Geometry check sheet. Reference: the model listing, model coordinates, mm. A direction names the side the tool comes from. Give positions to 0.01 mm unless a question says otherwise; leave off trailing zeros. Write each loop counter-clockwise with the first axis right and the second up, starting at its lowest first coordinate (ties: lowest second). Pieces come first, ordered by that corner, then holes. Notation, with made-up numbers: (48.25, 43.25) - (81.25, 43.25) arc R18 ccw to (81.25, 69.25) - close; hole circle Ø8 at (27.25, 29). An arc over 180 degrees is marked (long way). Write item = value, one per line. Start each with the question number.
(1) Section check C-C, the plane x = -46. Enter the section's corners in (y, z).
(2) Section check A-A, the plane y = 31.5. Enter the section's corners in (x, z).
(3) Section check D-D, the plane y = 37.5. Enter the section's corners in (x, z), plus the area to 3 significant figures.
(4) Section check B-B, the plane z = 2.65. Enter the section's corners in (x, y), plus the area to 3 significant figures.
(5) Depth check by flat-ended pin: pin 1 Ø1 at (y, z) = (36.5, 1) entering from -X; pin 2 Ø3 at (x, y) = (-38.33, 34.29) entering from +Z; pin 3 Ø1 at (x, z) = (-39.5, 3.5) entering from +Y. Enter the tip coordinate at first touch or a pass-through.
(6) Thickness scan on L1, parallel to X at y = 32.75, z = 2.05; L2, parallel to X at y = 33.25, z = 2.8; L3, parallel to Z at x = -35.5, y = 36.25. Record the ranges inside material, lowest first.
(7) Access from +Z, -Z, +X, -X, +Y, -Y to the whole of each face (thin tool, end or side, straight path). Record for faces 1 (the flat face through (-43, 34, 0)), 2 (the flat face through (-38, 34, 1)).
(8) Draft check along X on faces 3 (the cylindrical face through (-49.21, 32.47, 2.97)), 4 (the flat face through (-46, 32, 5)). Enter one of: pulls with the +X half, pulls with the -X half, needs draft (parallel to the pull), parting line crosses it, or undercut.
```python
from build123d import *

# Parameters (mm, degrees)
F0_R     = 3
F0_R_2   = 2
F1_DEPTH = 5
F2_DEPTH = 1
F3_DEPTH = 0.5


# Not quite as in the source:
# - a feature names something its author has since deleted; it is built from what else it names


with BuildPart() as f1:
    # F0 (on Top) → F1 (new body)
    with BuildSketch(Plane.XY):
        with Locations((-46.8270219862, 34.2949032784)):
            Circle(F0_R)
        with Locations((-46.8270219862, 34.2949032784)):
            Circle(F0_R_2, mode=Mode.SUBTRACT)
    extrude(amount=F1_DEPTH)

    # F0 (on Top) → F2 (join)
    with BuildSketch(Plane.XY):
        with BuildLine():
            ThreePointArc((-42.8347911995, 34.0457179145), (-42.8289647614, 34.1702500531), (-42.8270219862, 34.2949032784))
            ThreePointArc((-42.8270219862, 34.2949032784), (-42.8289647614, 34.4195565036), (-42.8347911995, 34.5440886422))
            ThreePointArc((-42.8347911995, 34.5440886422), (-50.8270219862, 34.2949032784), (-42.8347911995, 34.0457179145))
        make_face()
        with Locations((-46.8270219862, 34.2949032784)):
            Circle(F0_R, mode=Mode.SUBTRACT)
        with Locations((-46.8270219862, 34.2949032784)):
            Circle(F0_R_2)
    extrude(amount=F2_DEPTH)



with BuildPart() as f1b:
    # F0 (on Top) → F1, piece 2 (new body)
    with BuildSketch(Plane.XY):
        with Locations((-38.3270219862, 34.2949032784)):
            Circle(F0_R)
        with Locations((-38.3270219862, 34.2949032784)):
            Circle(F0_R_2, mode=Mode.SUBTRACT)
    extrude(amount=F1_DEPTH)

    # F0 (on Top) → F2, piece 2 (join)
    with BuildSketch(Plane.XY):
        with BuildLine():
            ThreePointArc((-34.3270219862, 34.2949032784), (-38.202368761, 38.2929605032), (-42.319252773, 34.5440886422))
            ThreePointArc((-42.319252773, 34.5440886422), (-42.3270219862, 34.2949032784), (-42.319252773, 34.0457179145))
            ThreePointArc((-42.319252773, 34.0457179145), (-38.202368761, 30.2968460535), (-34.3270219862, 34.2949032784))
        make_face()
        with Locations((-38.3270219862, 34.2949032784)):
            Circle(F0_R, mode=Mode.SUBTRACT)
        with Locations((-38.3270219862, 34.2949032784)):
            Circle(F0_R_2)
    extrude(amount=F2_DEPTH)


with BuildPart() as f1_1:
    add(f1.part)

    add(f1b.part)  # F3 merges F1b
    # F0 (on Top) → F3 (join)
    with BuildSketch(Plane.XY):
        with BuildLine():
            ThreePointArc((-42.8347911995, 34.5440886422), (-42.8289647614, 34.4195565036), (-42.8270219862, 34.2949032784))
            ThreePointArc((-42.8270219862, 34.2949032784), (-42.8289647614, 34.1702500531), (-42.8347911995, 34.0457179145))
            Line((-42.8347911995, 34.0457179145), (-42.319252773, 34.0457179145))
            ThreePointArc((-42.319252773, 34.0457179145), (-42.3270219862, 34.2949032784), (-42.319252773, 34.5440886422))
            Line((-42.319252773, 34.5440886422), (-42.8347911995, 34.5440886422))
        make_face()
    extrude(amount=F3_DEPTH)


solid = f1_1.part
```
Model answer:
q1.outline = (30.38, 0) - (38.21, 0) - (38.21, 1) - (37.18, 1) - (37.18, 5) - (36.12, 5) - (36.12, 1) - (32.47, 1) - (32.47, 5) - (31.41, 5) - (31.41, 1) - (30.38, 1) - close
q2.outline = (-49.69, 0) - (-43.97, 0) - (-43.97, 1) - (-45.74, 1) - (-45.74, 5) - (-47.92, 5) - (-47.92, 1) - (-49.69, 1) - close; (-41.19, 0) - (-35.47, 0) - (-35.47, 1) - (-37.24, 1) - (-37.24, 5) - (-39.42, 5) - (-39.42, 1) - (-41.19, 1) - close
q3.outline = (-49.22, 0) - (-44.43, 0) - (-44.43, 1) - (-49.22, 1) - close; (-40.72, 0) - (-35.93, 0) - (-35.93, 1) - (-40.72, 1) - close
q3.area = 9.57 mm²
q4.outline = circle Ø6 at (-46.83, 34.29); circle Ø6 at (-38.33, 34.29); hole circle Ø4 at (-46.83, 34.29); hole circle Ø4 at (-38.33, 34.29)
q4.area = 31.4 mm²
q5.pin_1 = -50.45
q5.pin_2 = 1
q5.pin_3 = 37.22
q6.L1 = -49.4 to -48.1, -45.56 to -44.26, -40.9 to -39.6, -37.06 to -35.76
q6.L2 = -49.64 to -48.53, -45.12 to -44.01, -41.14 to -40.03, -36.62 to -35.51
q6.L3 = 0 to 1
q7.face_1 = -Z, +X, -X, +Y, -Y
q7.face_2 = +Z
q8.face_3 = undercut
q8.face_4 = needs draft
